from build123d import *

# Parameters (mm, degrees)
SKETCH_1_W               = 59.2
SKETCH_1_H               = 89
SKETCH_1_R               = 1.6
EXTRUDE_1_DEPTH          = 6.5
SKETCH_2_W               = 29.5
SKETCH_2_H               = 30
EXTRUDE_2_DEPTH          = 10
SKETCH_3_W               = 5
SKETCH_3_H               = 30
EXTRUDE_3_DEPTH          = 39
SKETCH_4_R               = 2.75
CUT_EXTRUDE_1_DEPTH      = 3.2
CUT_EXTRUDE_2_DEPTH      = 100
CUT_EXTRUDE_2_DEPTH_BACK = 100
SKETCH_5_R               = 1.6
SKETCH_6_R               = 3
CUT_EXTRUDE_3_DEPTH      = 5.5
FILLET_1_R               = 3
FILLET_2_R               = 5
FILLET_5_R               = 1
FILLET_6_R               = 5
SKETCH_7_RX              = 20.824026905
SKETCH_7_RY              = 15.170998686
CUT_EXTRUDE_4_DEPTH      = 10


# Some blends are built 0.0001 mm under size
with BuildPart() as part:
    # 草图1 → 凸台-拉伸1 (new body)
    with BuildSketch(Plane.XY):
        with Locations((0, -7)):
            Rectangle(SKETCH_1_W, SKETCH_1_H)
        with Locations(Location((-23, -32.5, 0), (0, 0, 180))):
            Circle(SKETCH_1_R, mode=Mode.SUBTRACT)
        with Locations(Location((23, -32.5, 0), (0, 0, 180))):
            Circle(SKETCH_1_R, mode=Mode.SUBTRACT)
        with Locations(Location((23, 32.5, 0), (0, 0, 180))):
            Circle(SKETCH_1_R, mode=Mode.SUBTRACT)
        with Locations(Location((-23, 32.5, 0), (0, 0, 180))):
            Circle(SKETCH_1_R, mode=Mode.SUBTRACT)
    extrude(amount=EXTRUDE_1_DEPTH)

    # 草图2 → 凸台-拉伸2 (add)
    with BuildSketch(Plane(origin=(0, 0, 0), x_dir=(-1, 0, 0), z_dir=(0, 0, -1))):
        with Locations((0, 20.5)):
            Rectangle(SKETCH_2_W, SKETCH_2_H)
    extrude(amount=EXTRUDE_2_DEPTH)

    # 草图3 → 凸台-拉伸3 (add)
    with BuildSketch(Plane(origin=(0, 0, 0), x_dir=(-1, 0, 0), z_dir=(0, 0, -1))):
        with Locations((17.25, 20.5)):
            Rectangle(SKETCH_3_W, SKETCH_3_H)
        with Locations((-17.25, 20.5)):
            Rectangle(SKETCH_3_W, SKETCH_3_H)
    extrude(amount=EXTRUDE_3_DEPTH)

    # 草图4 → 切除-拉伸1 (cut)
    with BuildSketch(Plane(origin=(0, 0, 0), x_dir=(-1, 0, 0), z_dir=(0, 0, -1))):
        with Locations((23, -32.5)):
            Circle(SKETCH_4_R)
        with Locations((-23, -32.5)):
            Circle(SKETCH_4_R)
        with Locations((23, 32.5)):
            Circle(SKETCH_4_R)
        with Locations((-23, 32.5)):
            Circle(SKETCH_4_R)
    extrude(amount=-CUT_EXTRUDE_1_DEPTH, mode=Mode.SUBTRACT)

    # 草图5 → 切除-拉伸2 (cut, two sides: drawn at the far end of the back side and taken through both)
    with BuildSketch(Plane(origin=(0, 0, -10), x_dir=(-1, 0, 0), z_dir=(0, 0, -1)).offset(-CUT_EXTRUDE_2_DEPTH_BACK)):
        with Locations(Location((0, 32.2, 0), (0, 0, 180))):
            Circle(SKETCH_5_R)
        with Locations(Location((10, 8.5, 0), (0, 0, 180))):
            Circle(SKETCH_5_R)
        with Locations(Location((-10, 8.5, 0), (0, 0, 180))):
            Circle(SKETCH_5_R)
    extrude(amount=CUT_EXTRUDE_2_DEPTH + CUT_EXTRUDE_2_DEPTH_BACK, mode=Mode.SUBTRACT)

    # 草图6 → 切除-拉伸3 (cut)
    with BuildSketch(Plane.XY.offset(6.5)):
        with Locations((10, 8.5)):
            Circle(SKETCH_6_R)
        with Locations((-10, 8.5)):
            Circle(SKETCH_6_R)
        with Locations((0, 32.2)):
            Circle(SKETCH_6_R)
    extrude(amount=-CUT_EXTRUDE_3_DEPTH, mode=Mode.SUBTRACT)

    # 圆角1
    fillet_1_edges = [part.edges().sort_by_distance(p)[0] for p in [
        (29.6, -51.5, 3.25),
        (-29.6, -51.5, 3.25),
        (-29.6, 37.5, 3.25),
        (29.6, 37.5, 3.25),
    ]]
    fillet(fillet_1_edges, radius=FILLET_1_R)

    # 圆角2
    # the kernel refuses this fillet: 5 mm, written as the material it adds along each edge
    with BuildSketch(Plane(origin=(-19.75, 5.5, 0), x_dir=(0, -1, 0), z_dir=(1, 0, 0))) as fillet_2_piece_1:
        with BuildLine():
            CenterArc((FILLET_2_R, FILLET_2_R), FILLET_2_R, 180, 90)
            Line((0, FILLET_2_R), (0, 0))
            Line((0, 0), (FILLET_2_R, 0))
        make_face()
    extrude(amount=39.5)
    with BuildSketch(Plane(origin=(-19.75, 35.5, 0), x_dir=(-1, 0, 0), z_dir=(0, -1, 0))) as fillet_2_piece_2_section:
        with BuildLine():
            CenterArc((FILLET_2_R, FILLET_2_R), FILLET_2_R, 180, 90)
            Line((0, FILLET_2_R), (0, 0))
            Line((0, 0), (FILLET_2_R, 0))
        make_face()
    fillet_2_piece_2 = extrude(amount=30, mode=Mode.PRIVATE)
    fillet_2_piece_2 = fillet_2_piece_2 - Plane(origin=(-23, 32.5, -1.1830281), x_dir=(-1, 0, 0), z_dir=(0, 0, -1)) * Cylinder(2.75, 80, mode=Mode.PRIVATE)
    add(fillet_2_piece_2)
    with BuildSketch(Plane(origin=(19.75, 35.5, 0), x_dir=(1, 0, 0), z_dir=(0, -1, 0))) as fillet_2_piece_3_section:
        with BuildLine():
            CenterArc((FILLET_2_R, -FILLET_2_R), FILLET_2_R, 90, 90)
            Line((0, -FILLET_2_R), (0, 0))
            Line((0, 0), (FILLET_2_R, 0))
        make_face()
    fillet_2_piece_3 = extrude(amount=30, mode=Mode.PRIVATE)
    fillet_2_piece_3 = fillet_2_piece_3 - Plane(origin=(23, 32.5, -1.183032565), x_dir=(-1, 0, 0), z_dir=(0, 0, -1)) * Cylinder(2.75, 80, mode=Mode.PRIVATE)
    add(fillet_2_piece_3)
    with BuildSketch(Plane(origin=(-32.25, 5.5, 0), x_dir=(0, -1, 0), z_dir=(1, 0, 0))) as fillet_2_piece_4a_section:
        with BuildLine():
            CenterArc((FILLET_2_R, FILLET_2_R), FILLET_2_R, 180, 90)
            Line((0, FILLET_2_R), (0, 0))
            Line((0, 0), (FILLET_2_R, 0))
        make_face()
    fillet_2_piece_4a = extrude(amount=52, mode=Mode.PRIVATE)
    fillet_2_piece_4a = split(fillet_2_piece_4a, bisect_by=Plane(origin=(-29.6, 4.368024429, -1.131975571), z_dir=(1, 0, 0)), keep=Keep.TOP, mode=Mode.PRIVATE)
    fillet_2_piece_4a = split(fillet_2_piece_4a, bisect_by=Plane(origin=(-19.75, 4.368024429, -1.131975571), z_dir=(-1, 0, 0)), keep=Keep.TOP, mode=Mode.PRIVATE)
    with BuildSketch(Plane(origin=(-19.75, 35.5, 0), x_dir=(-1, 0, 0), z_dir=(0, -1, 0))) as fillet_2_piece_4b_section:
        with BuildLine():
            CenterArc((FILLET_2_R, FILLET_2_R), FILLET_2_R, 180, 90)
            Line((0, FILLET_2_R), (0, 0))
            Line((0, 0), (FILLET_2_R, 0))
        make_face()
    fillet_2_piece_4b = extrude(amount=42.5, mode=Mode.PRIVATE)
    fillet_2_piece_4b = split(fillet_2_piece_4b, bisect_by=Plane(origin=(-20.881975571, 5.5, -1.131975571), z_dir=(0, -1, 0)), keep=Keep.TOP, mode=Mode.PRIVATE)
    fillet_2_piece_4 = fillet_2_piece_4a & fillet_2_piece_4b
    add(fillet_2_piece_4)
    with BuildSketch(Plane(origin=(-19.75, 5.5, 0), x_dir=(0, -1, 0), z_dir=(1, 0, 0))) as fillet_2_piece_5a_section:
        with BuildLine():
            CenterArc((FILLET_2_R, FILLET_2_R), FILLET_2_R, 180, 90)
            Line((0, FILLET_2_R), (0, 0))
            Line((0, 0), (FILLET_2_R, 0))
        make_face()
    fillet_2_piece_5a = extrude(amount=52, mode=Mode.PRIVATE)
    fillet_2_piece_5a = split(fillet_2_piece_5a, bisect_by=Plane(origin=(29.6, 4.368024429, -1.131975571), z_dir=(-1, 0, 0)), keep=Keep.TOP, mode=Mode.PRIVATE)
    fillet_2_piece_5a = split(fillet_2_piece_5a, bisect_by=Plane(origin=(19.75, 4.368024429, -1.131975571), z_dir=(1, 0, 0)), keep=Keep.TOP, mode=Mode.PRIVATE)
    with BuildSketch(Plane(origin=(19.75, 35.5, 0), x_dir=(1, 0, 0), z_dir=(0, -1, 0))) as fillet_2_piece_5b_section:
        with BuildLine():
            CenterArc((FILLET_2_R, -FILLET_2_R), FILLET_2_R, 90, 90)
            Line((0, -FILLET_2_R), (0, 0))
            Line((0, 0), (FILLET_2_R, 0))
        make_face()
    fillet_2_piece_5b = extrude(amount=42.5, mode=Mode.PRIVATE)
    fillet_2_piece_5b = split(fillet_2_piece_5b, bisect_by=Plane(origin=(20.881975571, 5.5, -1.131975571), z_dir=(0, -1, 0)), keep=Keep.TOP, mode=Mode.PRIVATE)
    fillet_2_piece_5 = fillet_2_piece_5a & fillet_2_piece_5b
    add(fillet_2_piece_5)

    # 圆角5
    fillet_5_edges = [part.edges().sort_by_distance(p)[0] for p in [
        (-29.6, -7, 0),
        (29.6, -7, 0),
        (0, -51.5, 0),
        (0, 37.5, 0),
        (-28.721320344, -50.621320344, 0),
        (28.721320344, -50.621320344, 0),
        (28.721320344, 36.621320344, 0),
        (-28.721320344, 36.621320344, 0),
    ]]
    fillet(fillet_5_edges, radius=FILLET_5_R)

    # 圆角6
    fillet_6_edges = [part.edges().sort_by_distance(p)[0] for p in [
        (-17.25, 5.5, -39),
        (-19.75, 20.5, -39),
        (-17.25, 35.5, -39),
        (17.25, 35.5, -39),
        (19.75, 20.5, -39),
        (17.25, 5.5, -39),
    ]]
    fillet(fillet_6_edges, radius=FILLET_6_R - 0.0001)  # a hair under: the kernel refuses the full size

    # 草图7 → 切除-拉伸4 (cut)
    with BuildSketch(Plane.XY.offset(6.5)):
        with Locations(Location((0, -21.62670202), (0, 0, -90))):
            Ellipse(SKETCH_7_RX, SKETCH_7_RY)
    extrude(amount=-CUT_EXTRUDE_4_DEPTH, mode=Mode.SUBTRACT)


solid = part.part
Model file for the job. Use its own axes, mm. A direction names the side the tool comes from. Give positions to 0.01 mm unless a question says otherwise; leave off trailing zeros. Order: outer loops, then holes, each group sorted by start corner. A loop starts at its lowest first (then second) coordinate and runs counter-clockwise, first axis right, second up. Notation, with made-up numbers: M 48.25,-16 L 52.25,-16 A16 ccw 52.25,-2 Z; hole C 18,24 d5. An arc over 180 degrees is marked long. Put each result on its own line as item: value. Start each with the question number.
(1) Tool access for faces 1 (the face through (14.75, 20, -24)), 2 (the face through (19.75, 20, -20)), 3 (the face through (22, -34, 3.2)): list every direction of +Z, -Z, +X, -X, +Y, -Y with a clear straight run to the whole face (end or side of a thin tool).
(2) Drill centre lines: L1, parallel to Y at x = -23, z = 4.8; L2, parallel to Y at x = 23, z = 1; L3, parallel to X at y = 32.5, z = 5.1. Where is each one in solid material? Low to high. Write a range as [from, to].
(3) Band-saw the part on C-C on x = -23. Give the cut face in (y, z), then the cut area to 3 significant figures.
(4) Band-saw the part on D-D on z = -1. Give the cut face in (x, y), then the cut area to 3 significant figures.
(5) Pull direction X, two halves, no side cores. Call faces 4 (the face through (12.77, 7.35, 3.79)), 5 (the face through (0, 35.5, -9)), 6 (the face through (21.25, 18.24, -1.43)): released by +X, released by -X, zero draft, split by the parting line, or undercut.
(6) Pin check, flat tips, straight feed: pin 1 Ø5 at (x, y) = (0, 32.2) entering from +Z; pin 2 Ø6 at (y, z) = (26.5, -19.5) entering from +X; pin 3 Ø12 at (x, z) = (22, -34.5) entering from -Y; pin 4 Ø2.5 at (x, y) = (-23, -32.5) entering from -Z. Stop position of each tip, or through.
(7) Band-saw the part on A-A on z = -12.5. Give the cut face in (x, y), then the cut area to 3 significant figures.
Results below:
1. face 1: -Z, +Y, -Y
1. face 2: -Z, +X, +Y, -Y
1. face 3: -Z
2. L1: y = [-51.5, -34.1], [-30.9, 30.9], [34.1, 37.5]
2. L2: y = [-51.5, -35.25], [-29.75, 29.75], [35.25, 37.5]
2. L3: x = [-29.6, -24.6], [-21.4, -2.98], [2.98, 21.4], [24.6, 29.6]
3. outline: M -51.5,1 A1 ccw -50.5,0 L -35.25,0 L -35.25,3.2 L -34.1,3.2 L -34.1,6.5 L -51.5,6.5 Z; M -30.9,3.2 L -29.75,3.2 L -29.75,0 L 0.5,0 A5 cw 2.25,-0.32 L 29.75,-0.32 L 29.75,3.2 L 30.9,3.2 L 30.9,6.5 L -30.9,6.5 Z; M 34.1,3.2 L 35.25,3.2 L 35.25,-0.32 L 35.5,-0.32 L 35.5,0 L 36.5,0 A1 ccw 37.5,1 L 37.5,6.5 L 34.1,6.5 Z
3. area: 531 mm2
4. outline: M -21.75,3.5 L 21.75,3.5 L 21.75,30.05 A2.75 cw 21.75,34.95 L 21.75,35.5 L -21.75,35.5 L -21.75,34.95 A2.75 cw -21.75,30.05 Z; hole C -10,8.5 d3.2; hole C 0,32.2 d3.2; hole C 10,8.5 d3.2
4. area: 1,360 mm2
5. face 4: undercut
5. face 5: zero draft
5. face 6: released by +X
6. pin 1: stops at z = 1
6. pin 2: stops at x = 19.75
6. pin 3: stops at y = 5.5
6. pin 4: passes through
7. outline: M -19.75,5.5 L -14.75,5.5 L -14.75,35.5 L -19.75,35.5 Z; M 14.75,5.5 L 19.75,5.5 L 19.75,35.5 L 14.75,35.5 Z
7. area: 300 mm2
